Can you work these out from the model? Positions are in its coordinate system, mm. Coordinates: 2 decimals unless noted, no trailing zeros. Order: outer loops, then holes, each group sorted by start corner. A loop starts at its lowest first (then second) coordinate and runs counter-clockwise, first axis right, second up.
Autodesk Inventor part; units mm, degrees
ref_plane "YZ Plane" through (0, 0, 0) normal (1, 0, 0) x (0, 1, 0)
ref_plane "XZ Plane" through (0, 0, 0) normal (0, 1, 0) x (-1, 0, 0)
ref_plane "XY Plane" through (0, 0, 0) normal (0, 0, 1) x (1, 0, 0)
sketch "Sketch1" plane through (0, 0, 0) normal (0, 0, 1) x (1, 0, 0)
  line L0 (0, 0) -> (3.019, 0)
  line L1 (3.4, -0.381) -> (3.4, -0.6409)
  line L2 (0, -1.8) -> (0, 0)
  line L3 (0, -1.8) -> (2.2393, -1.8)
  line L4 (2.3663, -1.673) -> (2.3663, -1.4282)
  line L5 (0, -1.3716) -> (0, -1.8)
  arc A0 (3.4, -0.381) -> (3.019, 0) centre (3.019, -0.381) ccw
  line L6 (2.4387, -1.5299) -> (2.511, -1.5299)
  arc A1 (2.511, -1.5299) -> (3.4, -0.6409) centre (2.511, -0.6409) ccw
  arc A2 (2.2393, -1.8) -> (2.3663, -1.673) centre (2.2393, -1.673) ccw
  line L7 (2.4387, -1.5299) -> (2.4387, -1.4282)
  line L8 (2.4387, -1.4282) -> (2.3663, -1.4282)
  point P0 (3.4, 0)
  dimension "d2" = 0.381
  dimension "d3" = 0.889
  dimension "d4" = 0.127
revolve "Revolution1" add sketch "Sketch1" angle 360 about axis through (0, -1.8, 0) along (0, 1, 0)
properties part number "SuperCap_PAS614L" material "Silver"
1. Please list where these lines run through material, in increasing order: probe 1 along Y at (x, z) = (2.5, 0); probe 2 along Z at (x, y) = (-1.5, -0.4); probe 3 along Y at (x, z) = (-0.5, 3).
Completed:
probe 1: y = -1.53 to 0
probe 2: z = -3.05 to 3.05
probe 3: y = -1.35 to 0
2. Imagine slicing it at C-C on y = -0.5. Please give me the cut outline in (x, z), then the cut area to 3 significant figures.
Completed:
outline: circle Ø6.8 at (0, 0)
area: 36.3 mm2
3. Imagine slicing it at A-A on x = 0. Please give me the cut outline in (y, z), then the cut area to 3 significant figures.
Completed:
outline: (-1.8, -2.24) arc R0.13 ccw to (-1.67, -2.37) - (-1.43, -2.37) - (-1.43, -2.44) - (-1.53, -2.44) - (-1.53, -2.51) arc R0.89 ccw to (-0.64, -3.4) - (-0.38, -3.4) arc R0.38 ccw to (0, -3.02) - (0, 3.02) arc R0.38 ccw to (-0.38, 3.4) - (-0.64, 3.4) arc R0.89 ccw to (-1.53, 2.51) - (-1.53, 2.44) - (-1.43, 2.44) - (-1.43, 2.37) - (-1.67, 2.37) arc R0.13 ccw to (-1.8, 2.24) - close
area: 11.3 mm2
4. Imagine slicing it at B-B on z = 0. Please give me the cut outline in (x, y).
Completed:
outline: (-3.4, -0.64) arc R0.89 ccw to (-2.51, -1.53) - (-2.44, -1.53) - (-2.44, -1.43) - (-2.37, -1.43) - (-2.37, -1.67) arc R0.13 ccw to (-2.24, -1.8) - (2.24, -1.8) arc R0.13 ccw to (2.37, -1.67) - (2.37, -1.43) - (2.44, -1.43) - (2.44, -1.53) - (2.51, -1.53) arc R0.89 ccw to (3.4, -0.64) - (3.4, -0.38) arc R0.38 ccw to (3.02, 0) - (-3.02, 0) arc R0.38 ccw to (-3.4, -0.38) - close
5. Imagine slicing it at D-D on y = -1. Please give me the cut outline in (x, z), then the cut area to 3 significant figures.
Completed:
outline: circle Ø6.65 at (0, 0)
area: 34.7 mm2
